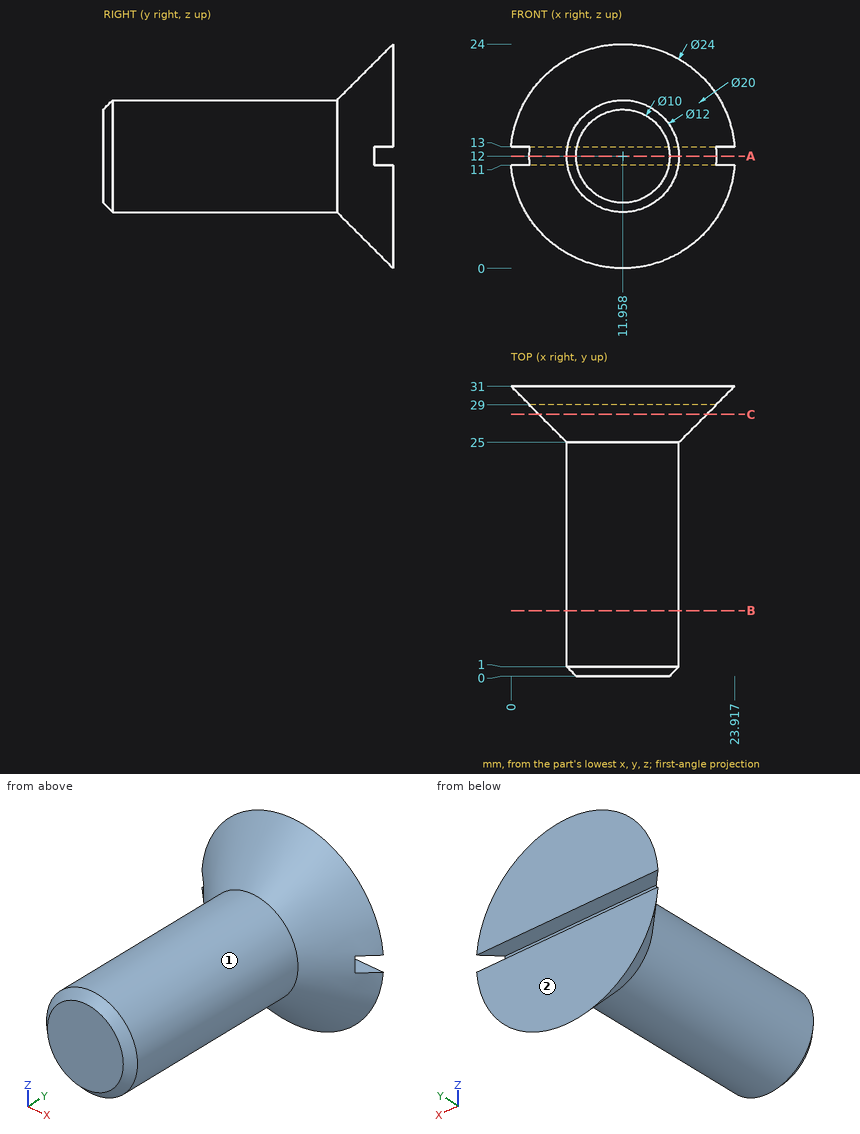
Here's the drawing with two shaded views (mm, measured from the low corner). I have some questions. A direction names the side the tool comes from. Give positions to 0.01 mm unless a question says otherwise; leave off trailing zeros. Loops run counter-clockwise (first coordinate to the right, second up) from the corner with the lowest first, then second, coordinate; pieces in that order, holes last. Notation, with made-up numbers: M -12.5,19 L 35.5,19 A7 ccw 35.5,31 Z; hole C -9,-23 d5. An arc over 180 degrees is marked long. Use one line per item in the form item = value. Start each with the question number.
(1) I want a section at B-B, the plane y = 7. Write out the boundary of the cut face in (x, z), and give its area (3 significant figures).
(2) I'm going to push flat-ended pins straight in: P1, Ø4, axis at y = 24.5, z = 8.5, coming from the -X side (1 decimal); P2, Ø5, axis at y = 17.5, z = 19, coming from the +X side (1 decimal); P3, Ø3, axis at x = 12, y = 15.5, coming from the -Z side. Where does each tip first touch, or does it pass through?
(3) Please list where these lines run through material, in increasing order: line 1 (Z direction, x = 8, y = 20.5); line 2 (X direction, y = 7, z = 11.75); line 3 (Z direction, x = 9, y = 21.5).
(4) I want a section at A-A, the plane z = 12. Write out the boundary of the cut face in (x, y), and give its area (3 significant figures).
(5) I want a section at C-C, the plane y = 28. Write out the boundary of the cut face in (x, z).
(6) On a 3-axis mill with a long thin cutter (end or side, diameter ignored), from which of +Z, -Z, +X, -X, +Y, -Y can I reach the whole of each face in a straight line? I mean the marked faces 1 and 2. Say none if no direction works.
Worked out:
q1.outline = C 11.96,12 d12
q1.area = 113 mm²
q2.P1 = 5.1
q2.P2 = 15.9
q2.P3 = 6
q3.line_1 = 7.49 to 16.51
q3.line_2 = 5.96 to 17.95
q3.line_3 = 6.78 to 17.22
q4.outline = M 1.96,29 L 5.96,25 L 5.96,1 L 6.96,0 L 16.96,0 L 17.96,1 L 17.96,25 L 21.96,29 Z
q4.area = 363 mm²
q5.outline = C 11.96,12 d18
q6.face_1 = -Y
q6.face_2 = +Z, -Z, +X, -X, +Y
